from build123d import *

# Parameters (mm, degrees)
F0_R      = 10
F1_DEPTH  = 5
F2_DEPTH  = 3
F3_R      = 3
F2_FACE_R = 7
F5_R      = 4.6788722556
F7_R      = 8
F7_R_2    = 4.6788722556
F8_DEPTH  = 2
F9_SIZE   = 1
F10_R     = 3.2686938503
F12_R     = 5.5
F14_SIZE  = 0.5
F16_DEPTH = 1
F17_DEPTH = 1
F19_W     = 2
F19_H     = 1.667086035
F20_DEPTH = 2
F18_W     = 2
F18_H     = 1.6840100288
F21_DEPTH = 2


with BuildPart() as f1:
    # F0 (on Top) → F1 (new body)
    with BuildSketch(Plane.XY):
        Circle(F0_R)
    extrude(amount=F1_DEPTH)

    # F2 (add): a face of the model
    f2_faces = [f1.faces().sort_by_distance(p)[0] for p in [
        (0, 0, 5),
    ]]
    extrude(f2_faces, amount=F2_DEPTH)

    # F3
    f3_edges = [f1.edges().sort_by_distance(p)[0] for p in [
        (-10, 0, 8),
    ]]
    fillet(f3_edges, radius=F3_R)

    # F2_face (on face) → F6 section 0
    with BuildSketch(Plane.XY.offset(8)):
        Circle(F2_FACE_R)
    # F5 (on offset) → F6 section 1
    with BuildSketch(Plane.XY.offset(28)):
        Circle(F5_R)
    loft()

    # F7 (on face) → F8 (join)
    with BuildSketch(Plane.XY.offset(28)):
        Circle(F7_R)
        Circle(F7_R_2, mode=Mode.SUBTRACT)
        Circle(F7_R_2)
    extrude(amount=F8_DEPTH)

    # F9
    f9_edges = [f1.edges().sort_by_distance(p)[0] for p in [
        (-8, 0, 30),
    ]]
    chamfer(f9_edges, length=F9_SIZE)

    # F10 (on face) → F13 section 0
    with BuildSketch(Plane.XY.offset(30)):
        Circle(F10_R)
    # F12 (on offset) → F13 section 1
    with BuildSketch(Plane.XY.offset(40)):
        Circle(F12_R)
    loft()

    # F14
    f14_edges = [f1.edges().sort_by_distance(p)[0] for p in [
        (-5.5, 0, 40),
    ]]
    chamfer(f14_edges, length=F14_SIZE)

    # F15 (on Front) → F16 (join)
    with BuildSketch(Plane.XZ):
        Polygon((-1.25, 45.55928049), (-1.25, 39.6955995162), (1.1311062619, 39.6955995162), (1.25, 39.6955995162), (1.25, 45.55928049), align=None)
    extrude(amount=F16_DEPTH)

    # F17 (add): a face of the model
    f17_faces = [f1.faces().sort_by_distance(p)[0] for p in [
        (0, 0, 42.779640245),
    ]]
    extrude(f17_faces, amount=F17_DEPTH)

    # F19 (on face) → F20 (join)
    with BuildSketch(Plane.YZ.offset(1.25)):
        with Locations((0, 42.681613937)):
            Rectangle(F19_W, F19_H)
    extrude(amount=F20_DEPTH)

    # F18 (on face) → F21 (join)
    with BuildSketch(Plane(origin=(-1.25, 0, 0), x_dir=(0, -1, 0), z_dir=(-1, 0, 0))):
        with Locations((0, 42.6668860018)):
            Rectangle(F18_W, F18_H)
    extrude(amount=F21_DEPTH)


solid = f1.part
The listing builds one solid part. Answer for the finished solid, in the listing's coordinates (mm). A direction names the side the tool comes from. Give positions to 0.01 mm unless a question says otherwise; leave off trailing zeros. Loops run counter-clockwise (first coordinate to the right, second up) from the corner with the lowest first, then second, coordinate; pieces in that order, holes last. Notation, with made-up numbers: (37.5, 47.5) - (93.5, 47.5) arc R13 ccw to (93.5, 61.5) - close; hole circle Ø9 at (-32, 77.25). An arc over 180 degrees is marked (long way). Write each question's results on one line, items separated by ' | '.
1. Consider probe 1 along Z at (x, y) = (2.5, -0.25); probe 2 along X at (y, z) = (0.5, 43); probe 3 along X at (y, z) = (0.75, 28.5). Determine where each line is inside the solid, lowest interval first. Write a range as from..to.
Resolved:
probe 1: z = 0..40, 41.85..43.52 | probe 2: x = -3.25..3.25 | probe 3: x = -7.96..7.96
2. Find section B-B, the plane x = 0. Write down the section's boundary in (y, z).
Resolved:
outline: (-10, 0) - (10, 0) - (10, 5) arc R3 ccw to (7, 8) - (4.68, 28) - (8, 28) - (8, 29) - (7, 30) - (3.27, 30) - (5.39, 39.51) - (5, 40) - (1, 40) - (1, 45.56) - (-1, 45.56) - (-1, 40) - (-5, 40) - (-5.39, 39.51) - (-3.27, 30) - (-7, 30) - (-8, 29) - (-8, 28) - (-4.68, 28) - (-7, 8) arc R3 ccw to (-10, 5) - close
3. Find section C-C, the plane z = 38.5. Write down the section's boundary in (x, y).
Resolved:
outline: circle Ø10.33 at (0, 0)
4. Which of the six approach directions +Z, -Z, +X, -X, +Y, -Y give full straight-line access (tool end or side, diameter ignored) to faces 4 (the face through (-0.758, 5.774, 18.14)), 5 (the face through (-3.25, 0, 43)), 6 (the face through (-1.73, -7.81, 28.49)), 7 (the face through (1.25, 0, 45))?
Resolved:
face 4: none | face 5: +Z, -X, +Y, -Y | face 6: +Z | face 7: +Z, +X, +Y, -Y
5. Find section A-A, the plane z = 4. Write down the section's boundary in (x, y), then the cut area to 3 significant figures.
Resolved:
outline: circle Ø20 at (0, 0) | area: 314 mm^2
6. For a pull along Z with two mould halves and no side action, classify faces 1 (the face through (1.25, 0, 41)), 2 (the face through (0, 1, 43)), 3 (the face through (2, 0, 43.515)) as +Z half, -Z half, draft (parallel to the pull), parting line (faces both ways), or undercut.
Resolved:
face 1: undercut | face 2: draft | face 3: +Z half
7. Flat-ended cylindrical pins translate along their axes: P1, Ø5, axis at x = 4.5, y = -5, coming from the +Z side; P2, Ø5, axis at y = 0, z = 15.5, coming from the +X side; P3, Ø5, axis at x = 3.5, y = 7.5, coming from the +Z side. Find the tip coordinate at first contact, or state that the pin passes through.
Resolved:
P1: stops at z = 40 | P2: stops at x = 6.42 | P3: stops at z = 30
